from build123d import *

# Parameters (mm, degrees)
SKETCH1_W           = 3
SKETCH1_H           = 1
BOSS_EXTRUDE1_DEPTH = 2.5
SKETCH2_R           = 0.5
BOSS_EXTRUDE2_DEPTH = 20
BOSS_EXTRUDE3_START = 1
SKETCH3_R           = 0.5
BOSS_EXTRUDE3_DEPTH = 1


with BuildPart() as part:
    # Sketch1 → Boss-Extrude1 (new body)
    with BuildSketch(Plane(origin=(0, 0, 0), x_dir=(1, 0, 0), z_dir=(0, 1, 0))):
        Rectangle(SKETCH1_W, SKETCH1_H)
    extrude(amount=BOSS_EXTRUDE1_DEPTH)

    # Sketch2 → Boss-Extrude2 (add)
    with BuildSketch(Plane(origin=(0, 2.5, 0), x_dir=(1, 0, 0), z_dir=(0, 1, 0))):
        with Locations(Location((0, 0, 0), (0, 0, 270))):
            Circle(SKETCH2_R)
    extrude(amount=BOSS_EXTRUDE2_DEPTH)

    # Sketch3 → Boss-Extrude3 (add)
    with BuildSketch(Plane.XZ.offset(BOSS_EXTRUDE3_START)):
        with Locations(Location((0, 0, 0), (0, 0, 90))):
            Circle(SKETCH3_R)
    extrude(amount=-BOSS_EXTRUDE3_DEPTH)


solid = part.part
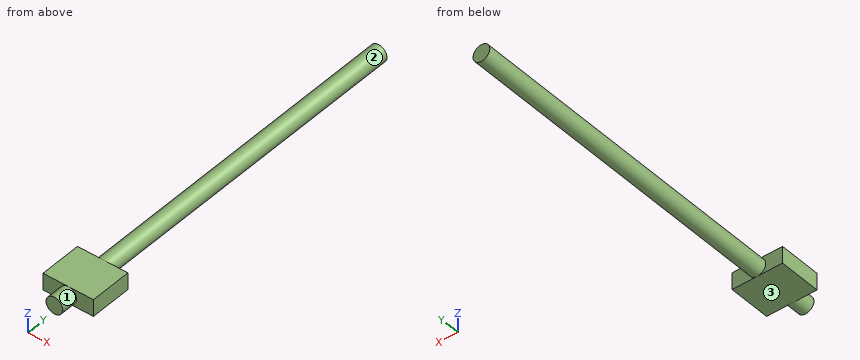
Read the model definition and answer for the solid it produces. Units are mm, in the model's axes. Face numbers are marked on the shaded views. A direction names the side the tool comes from. Coordinates: 2 decimals unless noted, no trailing zeros. Loops run counter-clockwise (first coordinate to the right, second up) from the corner with the lowest first, then second, coordinate; pieces in that order, holes last.
Q1. Consider probe 1 along Y at (x, z) = (0.55, -0.1); probe 2 along X at (y, z) = (19.25, 0); probe 3 along Z at (x, y) = (0.1, 6.5). Determine where each line is inside the solid, lowest interval first.
Q2. The part is cut by section B-B on y = 12.75. Write down the section's boundary in (x, z).
Q3. Which of the six approach directions +Z, -Z, +X, -X, +Y, -Y give full straight-line access (tool end or side, diameter ignored) to the marked faces 1, 2 and 3?
Q4. Each of these flat-tipped pins is pushed along its axis until it touches: pin 1 Ø0.5 at (x, z) = (1, 0) entering from -Y; pin 2 Ø1 at (x, y) = (0.5, 11) entering from -Z. Where does it stop, or does it pass through?
Q5. The part is cut by section A-A on z = 0. Write down the section's boundary in (x, y), and give its area (3 significant figures).
Results below:
1. probe 1: y = 0 to 2.5
1. probe 2: x = -0.5 to 0.5
1. probe 3: z = -0.49 to 0.49
2. outline: circle Ø1 at (0, 0)
3. face 1: -Y
3. face 2: +Y
3. face 3: -Z, +X, -X, +Y, -Y
4. pin 1: stops at y = 0
4. pin 2: stops at z = -0.5
5. outline: (-1.5, 0) - (-0.5, 0) - (-0.5, -1) - (0.5, -1) - (0.5, 0) - (1.5, 0) - (1.5, 2.5) - (0.5, 2.5) - (0.5, 22.5) - (-0.5, 22.5) - (-0.5, 2.5) - (-1.5, 2.5) - close
5. area: 28.5 mm2
